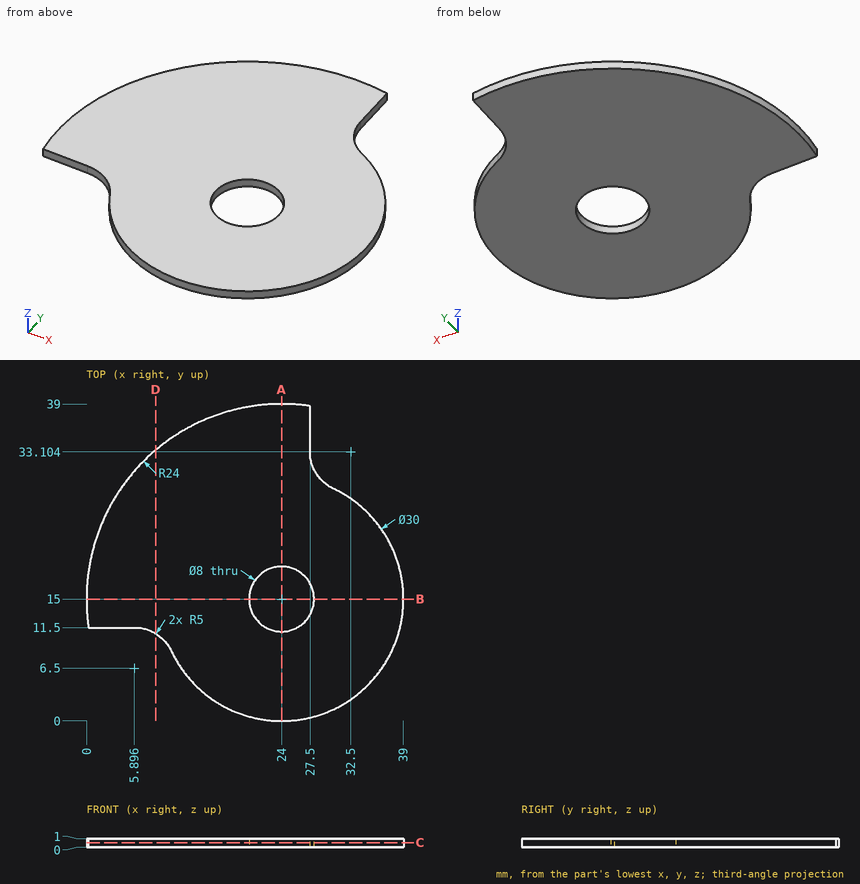
Job drawing, mm, ordinate dimensions from the low corner. One solid piece. Round coordinates to 2 decimals unless told otherwise and drop trailing zeros. Loops run counter-clockwise (first coordinate to the right, second up) from the corner with the lowest first, then second, coordinate; pieces in that order, holes last.
(1) Cut at B-B (y = 15). Give the cut face in (x, z), plus the area to 3 significant figures.
(2) Cut at A-A (x = 24). Give the cut face in (y, z).
(3) Wall check: line 1 along Y through (x, z) = (24, 0.6); line 2 along X through (y, z) = (12.5, 0.5); line 3 along Y through (x, z) = (20.5, 0.95) (1 decimal). Give the ranges that are in metal, low to high.
(4) Cut at C-C (z = 0.55). Give the cut face in (x, y) (1 decimal).
(5) Cut at D-D (x = 8.5). Give the cut face in (y, z).
(6) Drop flat-ended pins along their axis: pin 1 (0.5 mm diameter, centred on x = 3, z = 0.5, fed in from -Y); pin 2 (0.5 mm diameter, centred on y = 37, z = 0.5, fed in from +X). Give the stop position or say it passes through.
Findings below:
1. outline: (0, 0) - (20, 0) - (20, 1) - (0, 1) - close; (28, 0) - (39, 0) - (39, 1) - (28, 1) - close
1. area: 31.0 mm2
2. outline: (0, 0) - (11, 0) - (11, 1) - (0, 1) - close; (19, 0) - (39, 0) - (39, 1) - (19, 1) - close
3. line 1: y = 0 to 11, 19 to 39
3. line 2: x = 0.13 to 20.88, 27.12 to 38.79
3. line 3: y = 0.4 to 13.1, 16.9 to 38.7
4. outline: (0.3, 11.5) - (5.9, 11.5) arc R5 cw to (10.4, 8.6) arc R15 ccw (long way) to (30.4, 28.6) arc R5 cw to (27.5, 33.1) - (27.5, 38.7) arc R24 ccw to start; hole circle Ø8 at (24, 15)
5. outline: (10.77, 0) - (33.32, 0) - (33.32, 1) - (10.77, 1) - close
6. pin 1: stops at y = 11.5
6. pin 2: stops at x = 27.5
